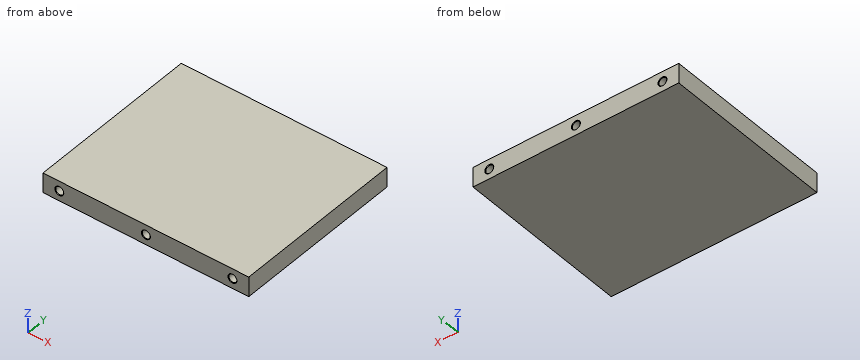
from build123d import *

# Parameters (mm, degrees)
SKETCH1_W           = 208
SKETCH1_H           = 20
BOSS_EXTRUDE1_DEPTH = 175
SKETCH2_R           = 4
CUT_EXTRUDE1_DEPTH  = 12
CHAMFER1_SIZE       = 0.5


with BuildPart() as part:
    # Sketch1 → Boss-Extrude1 (new body)
    with BuildSketch(Plane(origin=(0, 0, -58), x_dir=(1, 0, 0), z_dir=(0, 1, 0))):
        with Locations((0, -58)):
            Rectangle(SKETCH1_W, SKETCH1_H)
    extrude(amount=BOSS_EXTRUDE1_DEPTH)

    # Sketch2 → Cut-Extrude1 (cut)
    with BuildSketch(Plane(origin=(0, 175, 0), x_dir=(1, 0, 0), z_dir=(0, 1, 0))):
        Circle(SKETCH2_R)
        with Locations((-87.5, 0)):
            Circle(SKETCH2_R)
        with Locations((87.5, 0)):
            Circle(SKETCH2_R)
    cut_extrude1 = extrude(amount=-CUT_EXTRUDE1_DEPTH, mode=Mode.SUBTRACT)

    # Mirror6: Cut-Extrude1 across plane
    add(cut_extrude1.mirror(Plane.ZX.offset(87.5)), mode=Mode.SUBTRACT)

    # Chamfer1
    chamfer1_edges = [part.edges().sort_by_distance(p)[0] for p in [
        (83.5, 175, 0),
        (-91.5, 175, 0),
        (-4, 175, 0),
        (83.5, 0, 0),
        (-91.5, 0, 0),
        (-4, 0, 0),
    ]]
    chamfer(chamfer1_edges, length=CHAMFER1_SIZE)


solid = part.part
Geometry check sheet. Reference: the model listing, model coordinates, mm. Give positions to 0.01 mm unless a question says otherwise; leave off trailing zeros. Write each loop counter-clockwise with the first axis right and the second up, starting at its lowest first coordinate (ties: lowest second). Pieces come first, ordered by that corner, then holes. Notation, with made-up numbers: (38.25, 64) - (78.25, 64) arc R19 cw to (78.25, 98) - close; hole circle Ø3 at (45.5, 58). An arc over 180 degrees is marked (long way). Put each result on its own line as item: value.
1. Go/stop test with flat-tipped pins: pin 1 (6.5 mm diameter, centred on x = 0, z = 0, fed in from +Y); pin 2 (5 mm diameter, centred on x = -87.5, z = 0, fed in from -Y). Record where each tip stops, or that it passes through.
Ans:
pin 1: stops at y = 163
pin 2: stops at y = 12
2. Thickness scan on line 1 (X direction, y = 171.5, z = 0); line 2 (Z direction, x = 0, y = 165); line 3 (Z direction, x = -85, y = 164). Record the ranges inside material, lowest first.
Ans:
line 1: x = -104 to -91.5, -83.5 to -4, 4 to 83.5, 91.5 to 104
line 2: z = -10 to -4, 4 to 10
line 3: z = -10 to -3.12, 3.12 to 10
3. Sectioned sample at A-A, the plane x = -87.5. Enter the section's corners in (y, z), plus the area to 3 significant figures.
Ans:
outline: (0, -10) - (175, -10) - (175, -4.5) - (174.5, -4) - (163, -4) - (163, 4) - (174.5, 4) - (175, 4.5) - (175, 10) - (0, 10) - (0, 4.5) - (0.5, 4) - (12, 4) - (12, -4) - (0.5, -4) - (0, -4.5) - close
area: 3,310 mm²
